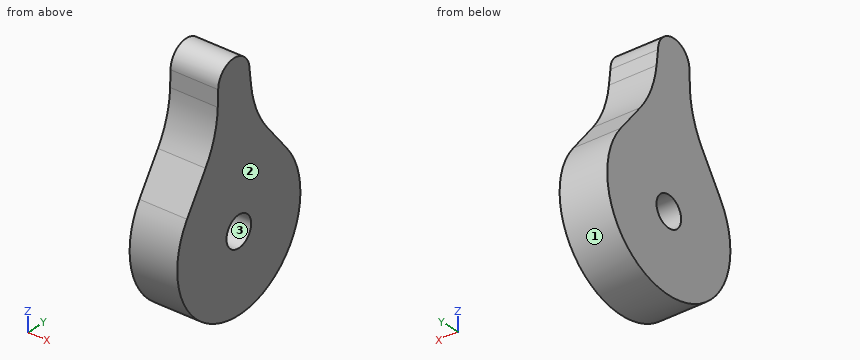
from build123d import *

# Parameters (mm, degrees)
SKETCH2_R           = 8
SKETCH2_R_2         = 1.6
BOSS_EXTRUDE1_DEPTH = 5
BOSS_EXTRUDE2_START = -5
BOSS_EXTRUDE2_DEPTH = 5
FILLET1_R           = 10
FILLET2_R           = 10


with BuildPart() as part:
    # Sketch2 → Boss-Extrude1 (new body)
    with BuildSketch(Plane(origin=(0, 0, 0), x_dir=(0, 0, -1), z_dir=(1, 0, 0))):
        Circle(SKETCH2_R)
        Circle(SKETCH2_R_2, mode=Mode.SUBTRACT)
    extrude(amount=BOSS_EXTRUDE1_DEPTH)

    # Sketch3 → Boss-Extrude2 (add)
    with BuildSketch(Plane(origin=(5, 0, 0), x_dir=(0, 0, -1), z_dir=(1, 0, 0)).offset(BOSS_EXTRUDE2_START)):
        with BuildLine():
            Line((-10.375290129, -2.83397632), (-4.331302353, -6.726055302))
            ThreePointArc((-4.331302353, -6.726055302), (-7.989266236, -0.414276496), (-5.003749355, 6.241994264))
            Line((-5.003749355, 6.241994264), (-10.375290129, 1.93602368))
            Line((-10.375290129, 1.93602368), (-14.796152799, 1.399716967))
            ThreePointArc((-14.796152799, 1.399716967), (-16.836152799, -0.640283033), (-14.796152799, -2.680283033))
            Line((-14.796152799, -2.680283033), (-10.375290129, -2.83397632))
        make_face()
    extrude(amount=BOSS_EXTRUDE2_DEPTH)

    # Fillet1
    fillet1_edges = [part.edges().sort_by_distance(p)[0] for p in [
        (2.5, 1.93602368, 10.375290129),
    ]]
    fillet(fillet1_edges, radius=FILLET1_R)

    # Fillet2
    fillet2_edges = [part.edges().sort_by_distance(p)[0] for p in [
        (2.5, -2.83397632, 10.375290129),
    ]]
    fillet(fillet2_edges, radius=FILLET2_R)


solid = part.part
Can you work these out from the model? Positions are in its coordinate system, mm. Face numbers are marked on the shaded views. Give positions to 0.01 mm unless a question says otherwise; leave off trailing zeros. Order: outer loops, then holes, each group sorted by start corner. A loop starts at its lowest first (then second) coordinate and runs counter-clockwise, first axis right, second up. Notation, with made-up numbers: (79.5, -18) - (88.5, -18) arc R22 ccw to (88.5, 19) - close; hole circle Ø4 at (-12, 54). An arc over 180 degrees is marked (long way). Write each question's results on one line, items separated by ' | '.
1) Suppose I cut it at A-A, the plane x = 3.5. Write out the boundary of the cut face in (y, z), then the cut area to 3 significant figures.
Final values:
outline: (-6.73, 4.33) arc R8 ccw (long way) to (6.24, 5) - (3.72, 8.15) arc R10 cw to (1.59, 13.2) - (1.4, 14.8) arc R2.04 ccw to (-2.68, 14.8) - (-2.74, 13.13) arc R10 cw to (-4.32, 8.06) - close; hole circle Ø3.2 at (0, 0) | area: 241 mm^2
2) Suppose I cut it at B-B, the plane z = 0. Write out the boundary of the cut face in (x, y), then the cut area to 3 significant figures.
Final values:
outline: (0, -8) - (5, -8) - (5, -1.6) - (0, -1.6) - close; (0, 1.6) - (5, 1.6) - (5, 8) - (0, 8) - close | area: 64.0 mm^2
3) Suppose I cut it at C-C, the plane y = 0. Write out the boundary of the cut face in (x, z).
Final values:
outline: (0, -8) - (5, -8) - (5, -1.6) - (0, -1.6) - close; (0, 1.6) - (5, 1.6) - (5, 16.73) - (0, 16.73) - close
4) If we mould it in two halves opening along Y, with no side actions, what happens to the marked faces 1, 2 and 3? For each: pulls with the +Y half, pulls with the -Y half, needs draft (parallel to the pull), parting line crosses it, or undercut.
Final values:
face 1: parting line crosses it | face 2: needs draft | face 3: undercut
5) Suppose I cut it at D-D, the plane y = 2. Write out the boundary of the cut face in (x, z), then the cut area to 3 significant figures.
Final values:
outline: (0, -7.75) - (5, -7.75) - (5, 11.35) - (0, 11.35) - close | area: 95.5 mm^2
6) Please list where these lines run through material, in increasing order: line 1 along Y through (x, z) = (1.05, 0); line 2 along Y through (x, z) = (2.05, 14.75); line 3 along Z through (x, y) = (4.5, 1). Write a range as [from, to].
Final values:
line 1: y = [-8, -1.6], [1.6, 8] | line 2: y = [-2.68, 1.41] | line 3: z = [-7.94, -1.25], [1.25, 16.01]
7) I'm going to push flat-ended pins straight in: pin 1 Ø3 at (y, z) = (-3, 8) entering from -X; pin 2 Ø1 at (x, y) = (3.5, -5) entering from -Z; pin 3 Ø1 at (x, y) = (4.5, 1) entering from +Z; pin 4 Ø3 at (x, z) = (4.5, -5.5) entering from +Y. Where does each tip first touch, or does it pass through?
Final values:
pin 1: stops at x = 0 | pin 2: stops at z = -6.61 | pin 3: stops at z = 16.49 | pin 4: stops at y = 6.93
